```python
from build123d import *

# Parameters (mm, degrees)
CHAMFER1_SIZE      = 0.508
CHAMFER2_SIZE      = 1.524
CUT_EXTRUDE1_DEPTH = 41.9448
FILLET1_R          = 0.762


with BuildPart() as part:
    # Sketch1 → Revolve1 (revolve)
    with BuildSketch(Plane.XY):
        with BuildLine():
            Line((0, 43.0022), (0, -24.9936))
            Line((0, -24.9936), (-7.9375, -24.9936))
            Line((-7.9375, -24.9936), (-7.9375, -3.81))
            Line((-7.9375, -3.81), (-6.223, -3.81))
            Line((-6.223, -3.81), (-6.223, -1.27))
            ThreePointArc((-6.223, -1.27), (-6.594974388, -0.371974388), (-7.493, 0))
            Line((-7.493, 0), (-17.5006, 0))
            Line((-17.5006, 0), (-17.5006, 15.9512))
            Line((-17.5006, 15.9512), (-12.3825, 15.9512))
            Line((-12.3825, 15.9512), (-12.3825, 26.7462))
            ThreePointArc((-12.3825, 26.7462), (-9.652, 30.4038), (-12.3825, 34.0614))
            Line((-12.3825, 34.0614), (-12.3825, 37.7952))
            Line((-12.3825, 37.7952), (-7.1755, 43.0022))
            Line((-7.1755, 43.0022), (0, 43.0022))
        make_face()
    revolve(axis=Axis((0, -24.9936, 0), (0, -1, 0)))

    # Chamfer1
    chamfer1_edges = [part.edges().sort_by_distance(p)[0] for p in [
        (17.5006, 15.9512, 0),
        (17.5006, 0, 0),
    ]]
    chamfer(chamfer1_edges, length=CHAMFER1_SIZE)

    # Chamfer2
    chamfer2_edges = [part.edges().sort_by_distance(p)[0] for p in [
        (7.9375, -24.9936, 0),
    ]]
    chamfer(chamfer2_edges, length=CHAMFER2_SIZE)

    # Sketch2 → Cut-Extrude1 (cut, through all)
    with BuildSketch(Plane(origin=(0, 15.9512, 0), x_dir=(1, 0, 0), z_dir=(0, 1, 0))):
        with BuildLine():
            Line((-15.9512, 7.199320726), (-15.9512, -7.199320726))
            ThreePointArc((-15.9512, -7.199320726), (-17.5006, 0), (-15.9512, 7.199320726))
        make_face()
        with BuildLine():
            Line((15.9512, 7.199320726), (15.9512, -7.199320726))
            ThreePointArc((15.9512, -7.199320726), (17.5006, 0), (15.9512, 7.199320726))
        make_face()
    extrude(amount=-CUT_EXTRUDE1_DEPTH, mode=Mode.SUBTRACT)

    # Fillet1
    fillet1_edges = [part.edges().sort_by_distance(p)[0] for p in [
        (12.3825, 15.9512, 0),
    ]]
    fillet(fillet1_edges, radius=FILLET1_R)


solid = part.part
```
Input: part model. Units: mm. Frame: model coordinates. A direction names the side the tool comes from. Give positions to 0.01 mm unless a question says otherwise; leave off trailing zeros. Order: outer loops, then holes, each group sorted by start corner. A loop starts at its lowest first (then second) coordinate and runs counter-clockwise, first axis right, second up. Notation, with made-up numbers: M 31,75 L 88,75 A30 ccw 88,99 Z; hole C 72,13 d6. An arc over 180 degrees is marked long. Return JSON: item names as keys, results as strings.
Item 1: Access query for faces 1 (the conical face through (0.29, 15.81, 17.13)), 2 (the flat face through (5, -3.81, 4)), 3 (the cylindrical face through (1.72, -13.5, 7.75)). Directions: +Z, -Z, +X, -X, +Y, -Y. A direction counts if a zero-diameter tool reaches every point of the face in a straight line with its end or side. Return the directions, or none.
Solutions:
{"face 1": "+Z, +Y", "face 2": "none", "face 3": "-Y"}
Item 2: First-contact query: P1, Ø1, axis at y = 14, z = -12, coming from the -X side; P2, Ø1, axis at x = -8, y = 13, coming from the -Z side; P3, Ø10, axis at x = 4, y = 35, coming from the +Z side. Flat tips, straight axial feed; report the tip coordinate or a pass-through.
Solutions:
{"P1": "x = -13.19", "P2": "z = -15.81", "P3": "z = 12.38"}
Item 3: Ray query, probe 1 along Y at (x, z) = (-10, -1); probe 2 along Y at (x, z) = (-6, -13); probe 3 along Y at (x, z) = (-8, -3.5). Return the intervals inside material, ascending.
Solutions:
{"probe 1": "0 to 28.71, 32.1 to 40.13", "probe 2": "0 to 15.95", "probe 3": "0 to 41.45"}
Item 4: Cut plane D-D (y = 18). Return loops of the section in (x, z) (1 decimal).
Solutions:
{"outline": "C 0,0 d24.8"}
Item 5: Pull-direction query (Y, two-part tool) for faces 4 (the cylindrical face through (1.349, -2.522, 6.075)), 5 (the flat face through (5, 15.951, 13)), 6 (the cylindrical face through (-11.81, 21.8, -3.72)); classes: +Y half, -Y half, draft (parallel to the pull), parting line (faces both ways), or undercut.
Solutions:
{"face 4": "undercut", "face 5": "+Y half", "face 6": "draft"}
Item 6: Cut plane C-C (y = 3). Return loops of the section in (x, z), then the cut area to 3 significant figures.
Solutions:
{"outline": "M -15.95,-7.2 A17.5 ccw 15.95,-7.2 L 15.95,7.2 A17.5 ccw -15.95,7.2 Z", "area": "932 mm^2"}
Item 7: Cut plane B-B (z = 0). Return loops of the section in (x, y) (1 decimal), then the cut area to 3 significant figures.
Solutions:
{"outline": "M -16,0 L -7.5,0 A1.3 cw -6.2,-1.3 L -6.2,-3.8 L -7.9,-3.8 L -7.9,-23.5 L -6.4,-25 L 6.4,-25 L 7.9,-23.5 L 7.9,-3.8 L 6.2,-3.8 L 6.2,-1.3 A1.3 cw 7.5,0 L 16,0 L 16,16 L 13.1,16 A0.8 cw 12.4,16.7 L 12.4,26.7 A3.8 cw 12.4,34.1 L 12.4,37.8 L 7.2,43 L -7.2,43 L -12.4,37.8 L -12.4,34.1 A3.8 cw -12.4,26.7 L -12.4,16.7 A0.8 cw -13.1,16 L -16,16 Z", "area": "1,500 mm^2"}
